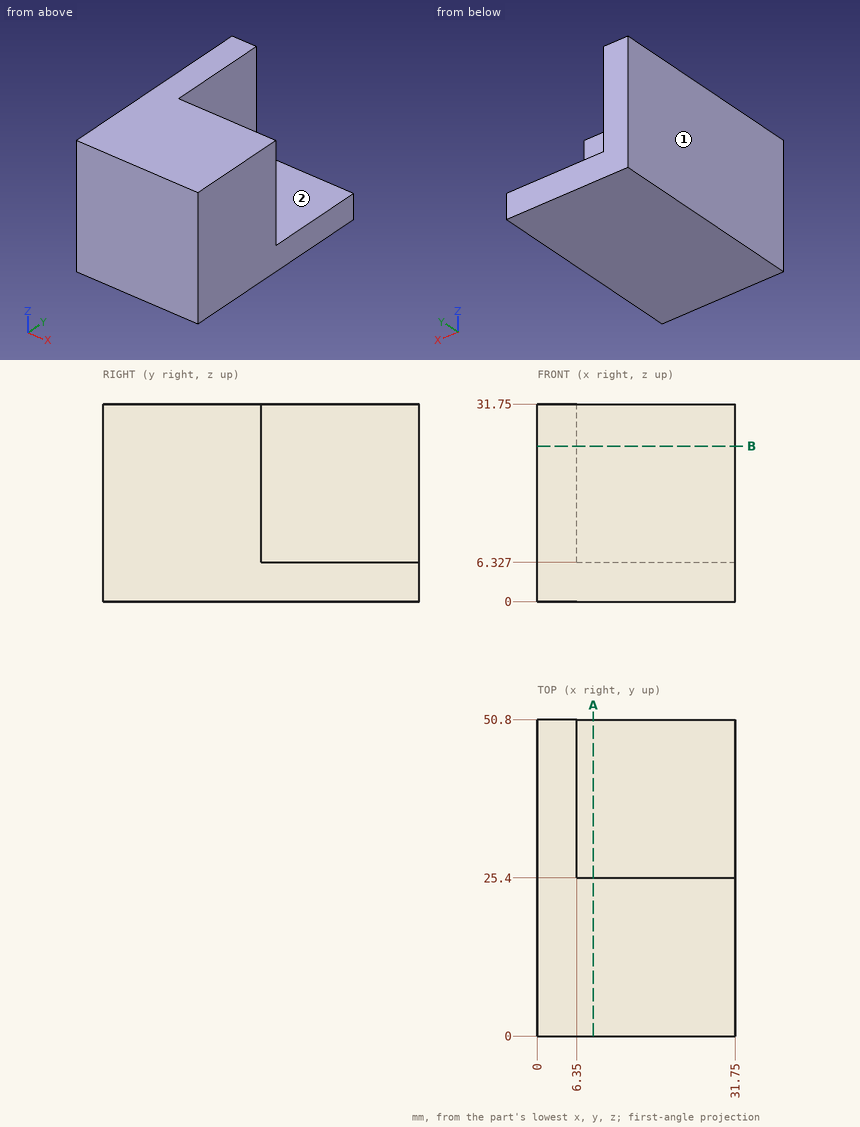
Here's the drawing with two shaded views (mm, measured from the low corner). I have some questions. A direction names the side the tool comes from. Give positions to 0.01 mm unless a question says otherwise; leave off trailing zeros. Order: outer loops, then holes, each group sorted by start corner. A loop starts at its lowest first (then second) coordinate and runs counter-clockwise, first axis right, second up. Notation, with made-up numbers: (47, 25.25) - (80, 25.25) arc R13 cw to (80, 49.25) - close; hole circle Ø2 at (-18.5, 76.5). An arc over 180 degrees is marked (long way). Write each question's results on one line, items separated by ' | '.
1) I'm going to push flat-ended pins straight in: pin 1 Ø7.5 at (x, z) = (20, 22.5) entering from +Y; pin 2 Ø1 at (x, y) = (23.5, 36.5) entering from +Z; pin 3 Ø7.5 at (y, z) = (33, 15.5) entering from +X. Where does each tip first touch, or does it pass through?
Final values:
pin 1: stops at y = 25.4 | pin 2: stops at z = 6.33 | pin 3: stops at x = 6.35
2) Please list where these lines run through material, in increasing order: line 1 along Y through (x, z) = (24.5, 25.5); line 2 along X through (y, z) = (39, 22.5); line 3 along Z through (x, y) = (19, 34). Write a range as [from, to].
Final values:
line 1: y = [0, 25.4] | line 2: x = [0, 6.35] | line 3: z = [0, 6.33]
3) On a 3-axis mill with a long thin cutter (end or side, diameter ignored), from which of +Z, -Z, +X, -X, +Y, -Y can I reach the whole of each face in a straight line? I mean the marked faces 1 and 2. Say none if no direction works.
Final values:
face 1: +Z, -Z, -X, +Y, -Y | face 2: +Z, +X, +Y
4) Suppose I cut it at B-B, the plane z = 25. Write out the boundary of the cut face in (x, y), then the cut area to 3 significant figures.
Final values:
outline: (0, 0) - (31.75, 0) - (31.75, 25.4) - (6.35, 25.4) - (6.35, 50.8) - (0, 50.8) - close | area: 968 mm^2
5) Suppose I cut it at A-A, the plane x = 9. Write out the boundary of the cut face in (y, z), then the cut area to 3 significant figures.
Final values:
outline: (0, 0) - (50.8, 0) - (50.8, 6.33) - (25.4, 6.33) - (25.4, 31.75) - (0, 31.75) - close | area: 967 mm^2
